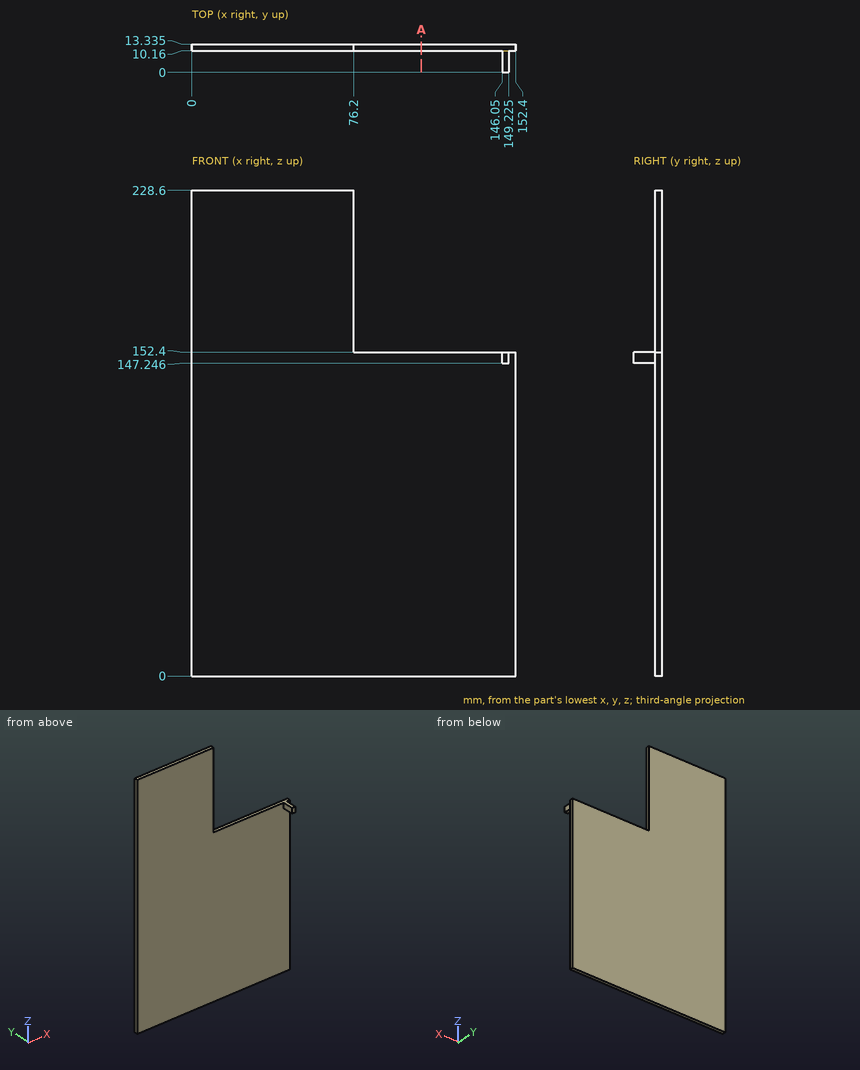
Print and shaded views of the part. All mm, measured from the part's lowest x, y and z. Round coordinates to 2 decimals unless told otherwise and drop trailing zeros. Write each loop counter-clockwise with the first axis right and the second up, starting at its lowest first coordinate (ties: lowest second). Pieces come first, ordered by that corner, then holes. Notation, with made-up numbers: M -33,-33.5 L 11,-33.5 A10 ccw 11,-19.5 Z; hole C 69.5,-36.5 d7. An arc over 180 degrees is marked long. Use a Markdown table: item, result. Add a question column.
1. Flat gauge pins, fed straight in: P1, Ø3.5, axis at y = 11.5, z = 177, coming from the +X side; P2, Ø3.5, axis at x = 148, y = 3.5, coming from the -Z side; P3, Ø5.5, axis at y = 3.5, z = 151, coming from the +X side (3 decimals). Where does each tip first touch, or does it go through?
2. Slice it at A-A on x = 108. Give the cut face in (y, z) (1 decimal).
3. Drill centre line: probe 1 along Y at (x, z) = (130, 56) (1 decimal). Where is it in solid material? Low to high.
Reply:
| question | item | result |
|---|---|---|
| 1 | P1 | stops at x = 76.2 |
| 1 | P2 | stops at z = 147.25 |
| 1 | P3 | stops at x = 149.225 |
| 2 | outline | M 10.2,0 L 13.3,0 L 13.3,152.4 L 10.2,152.4 Z |
| 3 | probe 1 | y = 10.2 to 13.3 |
